Design review of the part shown in the three views and the two pictorial views. Dimensions are in mm from the part's minimum x, y and z. A direction names the side the tool comes from. Coordinates: 2 decimals unless noted, no trailing zeros. Loops run counter-clockwise (first coordinate to the right, second up) from the corner with the lowest first, then second, coordinate; pieces in that order, holes last. Notation, with made-up numbers: (-19, -26) -> (0, -26) arc R11 ccw to (0, -13) -> close; hole circle Ø4 at (34, -25.5). An arc over 180 degrees is marked (long way). Use CSV: the item, a comma, the result in double quotes.
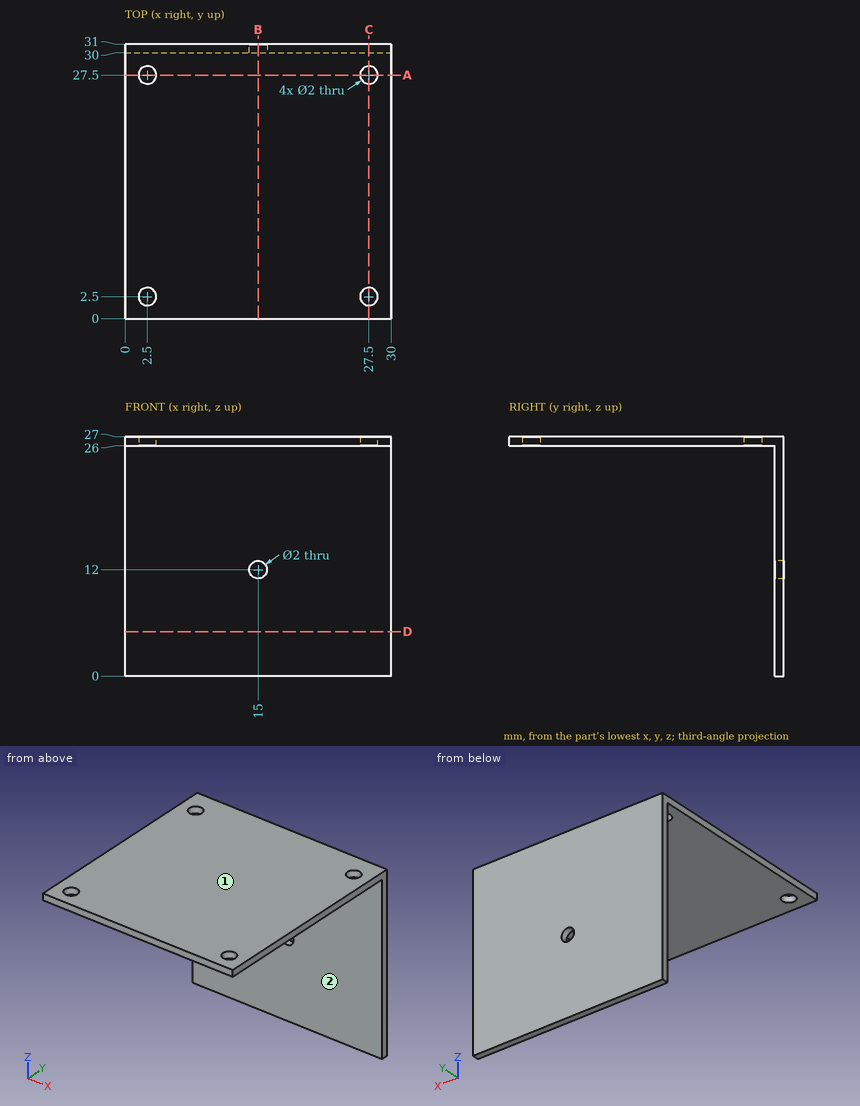
Item 1: Add section D-D (z = 5). Give the boundary of the cut face in (x, y).
Checked values:
outline,"(0, 30) -> (30, 30) -> (30, 31) -> (0, 31) -> close"
Item 2: Machinability: for the marked faces 1 and 2, which of the approach directions +Z, -Z, +X, -X, +Y, -Y give a long, thin tool a straight path to every point of the face, cutting with its end or side? Answer none if there is none.
Checked values:
face 1,"+Z, +X, -X, +Y, -Y"
face 2,"-Z, +X, -X, -Y"
Item 3: Add section A-A (y = 27.5). Give the boundary of the cut face in (x, z), then the cut area to 3 significant figures.
Checked values:
outline,"(0, 26) -> (1.5, 26) -> (1.5, 27) -> (0, 27) -> close; (3.5, 26) -> (26.5, 26) -> (26.5, 27) -> (3.5, 27) -> close; (28.5, 26) -> (30, 26) -> (30, 27) -> (28.5, 27) -> close"
area,"26.0 mm^2"
Item 4: Clearance check with flat-ended pins moving along their axes: pin 1 (2.5 mm diameter, centred on x = 2.5, y = 2.5, fed in from -Z); pin 2 (3 mm diameter, centred on x = 15, z = 12, fed in from -Y). State where each tip first meets the part, or that it passes through.
Checked values:
pin 1,"z = 26"
pin 2,"y = 30"
Item 5: Add section C-C (x = 27.5). Give the boundary of the cut face in (y, z), then the cut area to 3 significant figures.
Checked values:
outline,"(0, 26) -> (1.5, 26) -> (1.5, 27) -> (0, 27) -> close; (3.5, 26) -> (26.5, 26) -> (26.5, 27) -> (3.5, 27) -> close; (28.5, 26) -> (30, 26) -> (30, 0) -> (31, 0) -> (31, 27) -> (28.5, 27) -> close"
area,"53.0 mm^2"
Item 6: Add section B-B (x = 15). Give the boundary of the cut face in (y, z), then the cut area to 3 significant figures.
Checked values:
outline,"(0, 26) -> (30, 26) -> (30, 13) -> (31, 13) -> (31, 27) -> (0, 27) -> close; (30, 0) -> (31, 0) -> (31, 11) -> (30, 11) -> close"
area,"55.0 mm^2"
Item 7: To check wall thickness, follow line 1 along Y through (x, z) = (2.5, 26.2); line 2 along Z through (x, y) = (7.5, 5); line 3 along Y through (x, z) = (26, 21). State the ranges of each line that lie inside material, in increasing order.
Checked values:
line 1,"0 to 1.5, 3.5 to 26.5, 28.5 to 31"
line 2,"26 to 27"
line 3,"30 to 31"
